```python
from build123d import *

# Parameters (mm, degrees)
SKETCH1_R           = 10
BOSS_EXTRUDE1_DEPTH = 78
SKETCH2_R           = 2.8
CUT_EXTRUDE1_DEPTH  = 20
SKETCH3_R           = 3.6
CUT_EXTRUDE2_DEPTH  = 0.9
SKETCH4_R           = 1.8
CUT_EXTRUDE3_DEPTH  = 20
CHAMFER2_SIZE       = 2
CHAMFER2_SIZE2      = 0.352653961


with BuildPart() as part:
    # Sketch1 → Boss-Extrude1 (new body)
    with BuildSketch(Plane.XY):
        Circle(SKETCH1_R)
    extrude(amount=BOSS_EXTRUDE1_DEPTH)

    # Sketch2 → Cut-Extrude1 (cut)
    with BuildSketch(Plane.XY.offset(78)):
        Circle(SKETCH2_R)
    extrude(amount=-CUT_EXTRUDE1_DEPTH, mode=Mode.SUBTRACT)

    # Sketch3 → Cut-Extrude2 (cut)
    with BuildSketch(Plane.XY.offset(78)):
        Circle(SKETCH3_R)
    extrude(amount=-CUT_EXTRUDE2_DEPTH, mode=Mode.SUBTRACT)

    # Sketch4 → Cut-Extrude3 (cut)
    with BuildSketch(Plane(origin=(0, 0, 0), x_dir=(-1, 0, 0), z_dir=(0, 0, -1))):
        Circle(SKETCH4_R)
    extrude(amount=-CUT_EXTRUDE3_DEPTH, mode=Mode.SUBTRACT)

    # Chamfer2
    chamfer2_edges = [part.edges().sort_by_distance(p)[0] for p in [
        (1.8, 0, 0),
    ]]
    chamfer2_side = [part.faces().sort_by_distance(p)[0] for p in [
        (1.8, 0, 10),
    ]]
    chamfer(chamfer2_edges, length=CHAMFER2_SIZE, length2=CHAMFER2_SIZE2, reference=chamfer2_side[0])


solid = part.part
```
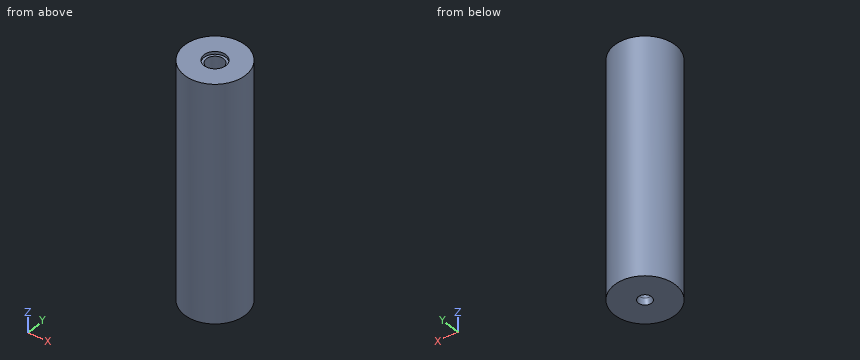
Input: part model. Units: mm. Frame: model coordinates. Coordinates: 2 decimals unless noted, no trailing zeros. Write each loop counter-clockwise with the first axis right and the second up, starting at its lowest first coordinate (ties: lowest second). Pieces come first, ordered by that corner, then holes. Notation, with made-up numbers: (60.5, 74) - (81.5, 74) arc R13 ccw to (81.5, 81) - close; hole circle Ø8 at (44, 5.25). An arc over 180 degrees is marked (long way). Put each result on its own line as item: value. Start each with the question number.
1) Cut plane D-D (z = 36). Return the cut outline in (x, y).
2) Cut plane A-A (z = 61). Return the cut outline in (x, y).
3) Cut plane B-B (y = 0). Return the cut outline in (x, z).
4) Contact query for flat-ended pins moving along their axis: pin 1 (8 mm diameter, centred on x = -6.5, z = 24, fed in from -Y); pin 2 (4 mm diameter, centred on x = 0, y = 0, fed in from +Z); pin 3 (6 mm diameter, centred on x = 3.5, z = 29.5, fed in from -Y). Output: stop coordinate, or through.
5) Ray query, L1, parallel to Y at x = 0, z = 14.5; L2, parallel to Y at x = 0, z = 73.25; L3, parallel to Z at x = 2.25, y = -1.25. Return the intervals inside material, ascending.
Resolved:
1. outline: circle Ø20 at (0, 0)
2. outline: circle Ø20 at (0, 0); hole circle Ø5.6 at (0, 0)
3. outline: (-10, 0) - (-2.15, 0) - (-1.8, 2) - (-1.8, 20) - (1.8, 20) - (1.8, 2) - (2.15, 0) - (10, 0) - (10, 78) - (3.6, 78) - (3.6, 77.1) - (2.8, 77.1) - (2.8, 58) - (-2.8, 58) - (-2.8, 77.1) - (-3.6, 77.1) - (-3.6, 78) - (-10, 78) - close
4. pin 1: stops at y = -9.68
4. pin 2: stops at z = 58
4. pin 3: stops at y = -9.99
5. L1: y = -10 to -1.8, 1.8 to 10
5. L2: y = -10 to -2.8, 2.8 to 10
5. L3: z = 0 to 58
